Design review of the part shown in the three views and the two pictorial views. Dimensions are in mm from the part's minimum x, y and z. Round coordinates to 2 decimals unless told otherwise and drop trailing zeros. Loops run counter-clockwise (first coordinate to the right, second up) from the corner with the lowest first, then second, coordinate; pieces in that order, holes last. Notation, with made-up numbers: M 48.5,65.25 L 75.5,65.25 A11 cw 75.5,77.25 Z; hole C 81.5,-25 d10. An arc over 180 degrees is marked long. Answer as CSV lines item,"result". Start each with the question number.
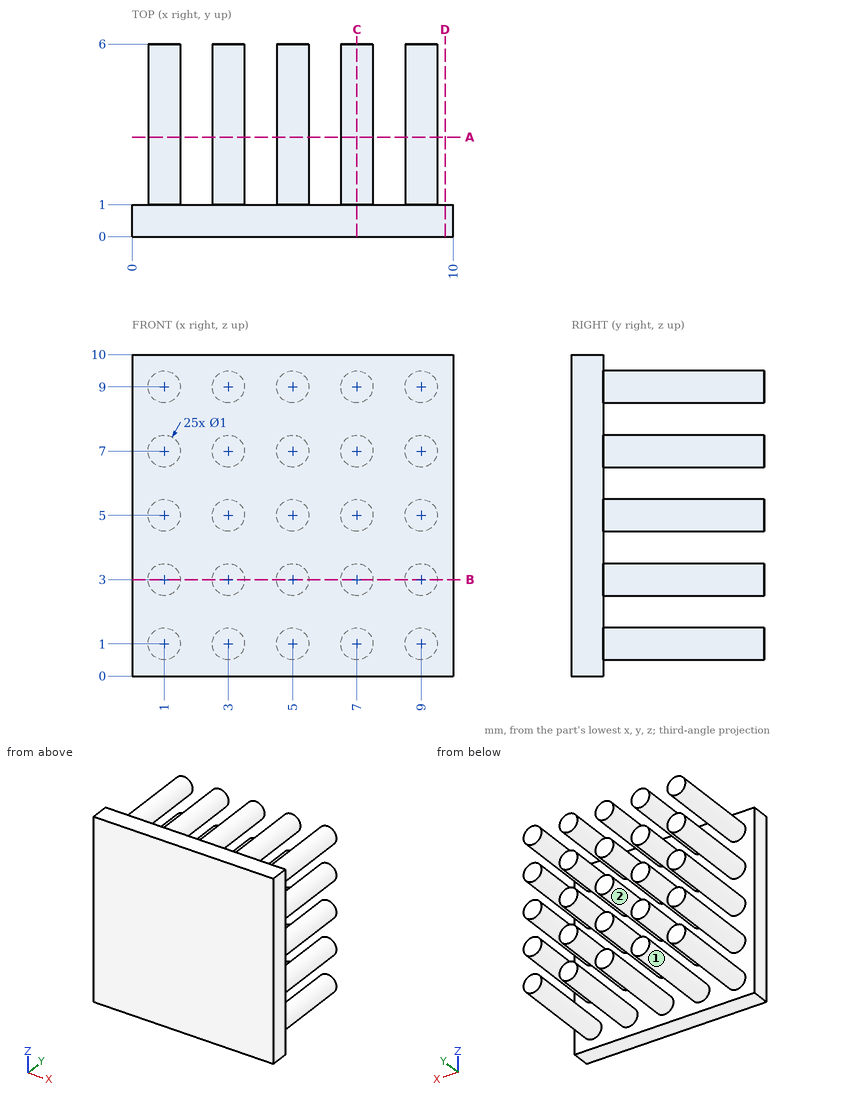
Item 1: To check wall thickness, follow line 1 (Z direction, x = 5, y = 2.15); line 2 (Z direction, x = 2.75, y = 3.5). State the ranges of each line that lie inside material, in increasing order.
Item 2: Consider section D-D, the plane x = 9.75. Write out the cut boundary in (y, z), then the cut area to 3 significant figures.
Item 3: Consider section B-B, the plane z = 3. Write out the cut boundary in (x, y), then the cut area to 3 significant figures.
Item 4: Insertion check: pin 1 Ø1.5 at (y, z) = (2.5, 5.5) entering from -X. The pin has a flat end and moves straight along its axis. Give the tip position at first contact, or say it passes through.
Item 5: The part is to be moulded in two halves that separate along Z. For the marked faces 1 and 2, say which applies: +Z half, -Z half, draft (parallel to the pull), parting line (faces both ways), or undercut.
Item 6: Consider section C-C, the plane x = 7. Write out the cut boundary in (y, z), then the cut area to 3 significant figures.
Item 7: Consider section A-A, the plane y = 3.1. Count the separate pieces of the cut face and the enclosed holes in it, then the cut area to 3 significant figures.
Found:
1,line 1,"z = 0.5 to 1.5, 2.5 to 3.5, 4.5 to 5.5, 6.5 to 7.5, 8.5 to 9.5"
1,line 2,"z = 0.57 to 1.43, 2.57 to 3.43, 4.57 to 5.43, 6.57 to 7.43, 8.57 to 9.43"
2,outline,"M 0,0 L 1,0 L 1,10 L 0,10 Z"
2,area,"10.0 mm^2"
3,outline,"M 0,0 L 10,0 L 10,1 L 9.5,1 L 9.5,6 L 8.5,6 L 8.5,1 L 7.5,1 L 7.5,6 L 6.5,6 L 6.5,1 L 5.5,1 L 5.5,6 L 4.5,6 L 4.5,1 L 3.5,1 L 3.5,6 L 2.5,6 L 2.5,1 L 1.5,1 L 1.5,6 L 0.5,6 L 0.5,1 L 0,1 Z"
3,area,"35.0 mm^2"
4,pin 1,"stops at x = 0.5"
5,face 1,"undercut"
5,face 2,"undercut"
6,outline,"M 0,0 L 1,0 L 1,0.5 L 6,0.5 L 6,1.5 L 1,1.5 L 1,2.5 L 6,2.5 L 6,3.5 L 1,3.5 L 1,4.5 L 6,4.5 L 6,5.5 L 1,5.5 L 1,6.5 L 6,6.5 L 6,7.5 L 1,7.5 L 1,8.5 L 6,8.5 L 6,9.5 L 1,9.5 L 1,10 L 0,10 Z"
6,area,"35.0 mm^2"
7,separate pieces,"25"
7,enclosed holes,"0"
7,area,"19.6 mm^2"
